CAD build for the part. Positions are in the model's coordinates, mm. Coordinates: 2 decimals unless noted, no trailing zeros. Write each loop counter-clockwise with the first axis right and the second up, starting at its lowest first coordinate (ties: lowest second). Pieces come first, ordered by that corner, then holes. Notation, with made-up numbers: M 25.5,67 L 30.5,67 A20 cw 30.5,84 Z; hole C 44.25,83 d3. An arc over 180 degrees is marked long. Answer as CSV lines item,"result". Start each with the question number.
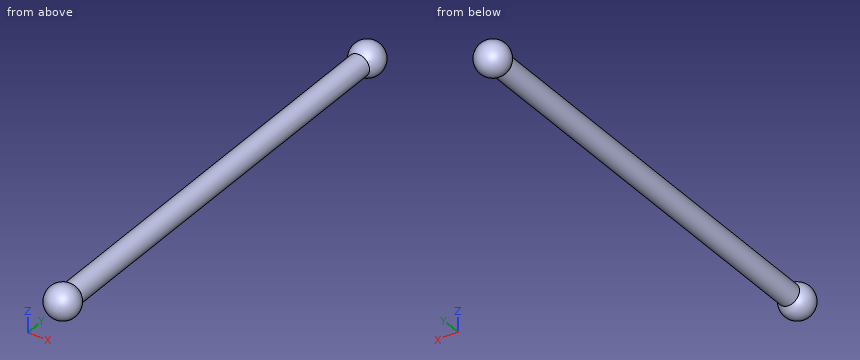
```python
from build123d import *

# Parameters (mm, degrees)
F0_R     = 1
F1_DEPTH = 20


with BuildPart() as f1:
    # F0 (on Front) → F1 (new body, symmetric)
    with BuildSketch(Plane.XZ):
        Circle(F0_R)
    extrude(amount=F1_DEPTH, both=True)

    # F2 (on Top) → F3 (revolve)
    with BuildSketch(Plane.XY):
        with BuildLine():
            Line((1.5, -20), (-1.5, -20))
            ThreePointArc((-1.5, -20), (0, -21.5), (1.5, -20))
        make_face()
    revolve(axis=Axis((0, -20, 0), (1, 0, 0)))

    # F4 (on Top) → F5 (revolve)
    with BuildSketch(Plane.XY):
        with BuildLine():
            Line((-1.5, 20), (1.5, 20))
            ThreePointArc((1.5, 20), (0, 21.5), (-1.5, 20))
        make_face()
    revolve(axis=Axis((0, 20, 0), (1, 0, 0)))


solid = f1.part
```
1) Band-saw the part on B-B, the plane y = 11.5. List the corners of the cut face in (x, z).
2) Band-saw the part on A-A, the plane x = 0. List the corners of the cut face in (y, z).
3) Pin check, flat tip, straight feed: P1, Ø1, axis at x = 0.5, y = 13, coming from the +Z side. Stop position of the tip, or through.
4) Band-saw the part on C-C, the plane z = 0. List the corners of the cut face in (x, y), plus the area to 3 significant figures.
5) Probe L1, parallel to X at y = -4, z = -0.05; L2, parallel to Y at x = -0.3, z = 1.3; L3, parallel to Z at x = 0.1, y = 1. List the from-to ranges inside material, lowest first. Write a range as [from, to].
Result sheet:
1,outline,"C 0,0 d2"
2,outline,"M -18.88,-1 L 18.88,-1 A1.5 ccw long 18.88,1 L -18.88,1 A1.5 ccw long Z"
3,P1,"stops at z = 1"
4,outline,"M -1,-18.88 A1.5 ccw long 1,-18.88 L 1,18.88 A1.5 ccw long -1,18.88 Z"
4,area,"88.6 mm²"
5,L1,"x = [-1, 1]"
5,L2,"y = [-20.69, -19.31], [19.31, 20.69]"
5,L3,"z = [-0.99, 0.99]"
